Verification items for this drawing (mm, ordinates from the low corner). A direction names the side the tool comes from. Coordinates: 2 decimals unless noted, no trailing zeros. Order: outer loops, then holes, each group sorted by start corner. A loop starts at its lowest first (then second) coordinate and runs counter-clockwise, first axis right, second up.
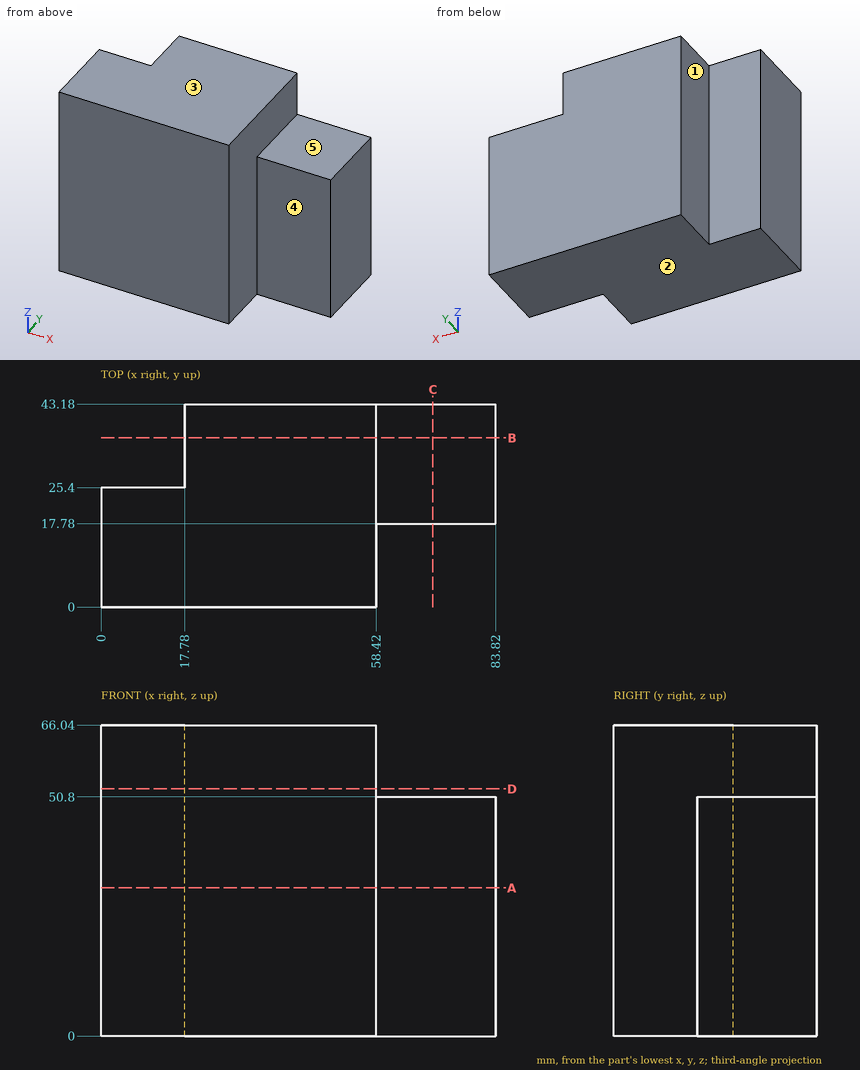
(1) Cross-section at D-D (z = 52.5). Enter the section's corners in (x, y).
Filled in:
outline: (0, 0) - (58.42, 0) - (58.42, 43.18) - (17.78, 43.18) - (17.78, 25.4) - (0, 25.4) - close
(2) Cross-section at A-A (z = 31.5). Enter the section's corners in (x, y), and give its area (3 significant figures).
Filled in:
outline: (0, 0) - (58.42, 0) - (58.42, 17.78) - (83.82, 17.78) - (83.82, 43.18) - (17.78, 43.18) - (17.78, 25.4) - (0, 25.4) - close
area: 2,850 mm2
(3) Cross-section at C-C (x = 70.5). Enter the section's corners in (y, z), and give its area (3 significant figures).
Filled in:
outline: (17.78, 0) - (43.18, 0) - (43.18, 50.8) - (17.78, 50.8) - close
area: 1,290 mm2
(4) Go/stop test with flat-tipped pins: P1, Ø4, axis at y = 23, z = 41, coming from the -X side; P2, Ø12.5, axis at x = 73, y = 25, coming from the +Z side; P3, Ø3, axis at x = 9, z = 46, coming from the +Y side; P4, Ø19.5, axis at y = 38.5, z = 29.5, coming from the -X side. Record where each tip stops, or that it passes through.
Filled in:
P1: stops at x = 0
P2: stops at z = 50.8
P3: stops at y = 25.4
P4: stops at x = 17.78
(5) Tool access check on the marked faces 1, 2, 3, 4 and 5. Record the directions out of +Z, -Z, +X, -X, +Y, -Y that give a thin tool (end or side, any length) a straight path to the whole face; none if there is none.
Filled in:
face 1: +Z, -Z, -X, +Y
face 2: -Z, +X, -X, +Y, -Y
face 3: +Z, +X, -X, +Y, -Y
face 4: +Z, -Z, +X, -Y
face 5: +Z, +X, +Y, -Y
(6) Thickness scan on probe 1 along X at (y, z) = (7, 63.5); probe 2 along Z at (x, y) = (78, 37); probe 3 along X at (y, z) = (28, 47). Record the ranges inside material, lowest first.
Filled in:
probe 1: x = 0 to 58.42
probe 2: z = 0 to 50.8
probe 3: x = 17.78 to 83.82
(7) Cross-section at B-B (y = 36). Enter the section's corners in (x, z).
Filled in:
outline: (17.78, 0) - (83.82, 0) - (83.82, 50.8) - (58.42, 50.8) - (58.42, 66.04) - (17.78, 66.04) - close
